Work out the finished part from the listing and answer in its coordinate system (mm). Face numbers are marked on the shaded views. A direction names the side the tool comes from. Round coordinates to 2 decimals unless told otherwise and drop trailing zeros. Loops run counter-clockwise (first coordinate to the right, second up) from the corner with the lowest first, then second, coordinate; pieces in that order, holes last. Notation, with made-up numbers: (-19.5, 66) -> (29.5, 66) arc R10 ccw to (29.5, 85) -> close; hole circle Ø3 at (8.25, 4.5). An arc over 180 degrees is marked (long way). Use one line per item in the form item = value.
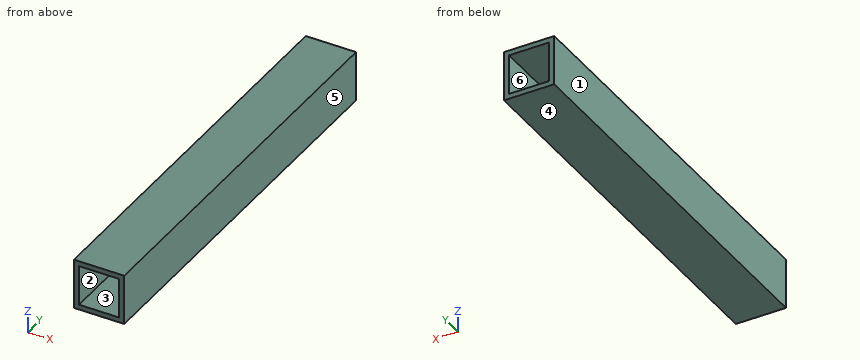
```python
from build123d import *

# Parameters (mm, degrees)
SKETCH_1_W      = 10
SKETCH_1_H      = 10
SKETCH_1_W_2    = 8
SKETCH_1_H_2    = 8
EXTRUDE_1_DEPTH = 80


with BuildPart() as part:
    # 草图1 → 凸台-拉伸1 (new body)
    with BuildSketch(Plane.XZ.offset(80)):
        with Locations((20, 0)):
            Rectangle(SKETCH_1_W, SKETCH_1_H)
        with Locations((20, 0)):
            Rectangle(SKETCH_1_W_2, SKETCH_1_H_2, mode=Mode.SUBTRACT)
    extrude(amount=-EXTRUDE_1_DEPTH)


solid = part.part
```
(1) Find section A-A, the plane x = 20. Write down the section's boundary in (y, z).
Completed:
outline = (-80, -5) -> (0, -5) -> (0, -4) -> (-80, -4) -> close; (-80, 4) -> (0, 4) -> (0, 5) -> (-80, 5) -> close
(2) Find section C-C, the plane y = -45. Write down the section's boundary in (x, z).
Completed:
outline = (15, -5) -> (25, -5) -> (25, 5) -> (15, 5) -> close; hole (16, -4) -> (24, -4) -> (24, 4) -> (16, 4) -> close
(3) Find section B-B, the plane z = -2.5. Write down the section's boundary in (x, y), then the cut area to 3 significant figures.
Completed:
outline = (15, -80) -> (16, -80) -> (16, 0) -> (15, 0) -> close; (24, -80) -> (25, -80) -> (25, 0) -> (24, 0) -> close
area = 160 mm2
(4) For the marked faces 1 and 2, determine the directions among +Z, -Z, +X, -X, +Y, -Y from which every point of the face is accessible in a straight line to the end or side of a thin tool.
Completed:
face_1 = +Z, -Z, -X, +Y, -Y
face_2 = +Y, -Y
(5) For a pull along X with two mould halves and no side action, classify the marked faces 3, 4, 5 and 6 as +X half, -X half, draft (parallel to the pull), parting line (faces both ways), or undercut.
Completed:
face_3 = undercut
face_4 = draft
face_5 = +X half
face_6 = undercut
(6) Given P1, Ø1.5, axis at x = 22.5, z = 0, coming from the -Y side, flat-ended and moving along its own axis, determine where the tip first touches the part or whether it passes through.
Completed:
P1 = through
(7) Consider L1, parallel to Z at x = 23.5, y = -15; L2, parallel to X at y = -48, z = 3. Determine where each line is inside the solid, lowest interval first.
Completed:
L1 = -5 to -4, 4 to 5
L2 = 15 to 16, 24 to 25
